from build123d import *

# Parameters (mm, degrees)
SKETCH1_W           = 105
SKETCH1_H           = 4
SKETCH1_W_2         = 2
SKETCH1_H_2         = 9.8
BOSS_EXTRUDE1_DEPTH = 12.5
SKETCH2_W           = 8
SKETCH2_H           = 10
SKETCH2_R           = 1.55
BOSS_EXTRUDE2_DEPTH = 2
SKETCH4_W           = 8
SKETCH4_H           = 10
SKETCH4_R           = 1.55
BOSS_EXTRUDE3_DEPTH = 2
SKETCH5_W           = 101
SKETCH5_H           = 2
CUT_EXTRUDE1_DEPTH  = 1.75
SKETCH6_W           = 101
SKETCH6_H           = 2
CUT_EXTRUDE2_DEPTH  = 1.75


with BuildPart() as part:
    # Sketch1 → Boss-Extrude1 (new body, symmetric)
    with BuildSketch(Plane(origin=(0, 0, 0), x_dir=(0, 0, -1), z_dir=(1, 0, 0))):
        Rectangle(SKETCH1_W, SKETCH1_H)
        Polygon((-52.5, 63.2), (-52.5, 2), (-48.5, 2), (-48.5, 63.2), (-50.5, 63.2), align=None)
        Polygon((48.5, 63.2), (48.5, 2), (52.5, 2), (52.5, 63.2), (50.5, 63.2), align=None)
        with Locations((-49.5, 68.1)):
            Rectangle(SKETCH1_W_2, SKETCH1_H_2)
        with Locations((49.5, 68.1)):
            Rectangle(SKETCH1_W_2, SKETCH1_H_2)
    extrude(amount=BOSS_EXTRUDE1_DEPTH, both=True)

    # Sketch2 → Boss-Extrude2 (add)
    with BuildSketch(Plane.XY.offset(-48.5)):
        with Locations((-16.5, 16)):
            Rectangle(SKETCH2_W, SKETCH2_H)
        with Locations((-16.5, 16)):
            Circle(SKETCH2_R, mode=Mode.SUBTRACT)
        with Locations((-16.5, 44)):
            Rectangle(SKETCH2_W, SKETCH2_H)
        with Locations((-16.5, 44)):
            Circle(SKETCH2_R, mode=Mode.SUBTRACT)
        with Locations((16.5, 16)):
            Rectangle(SKETCH2_W, SKETCH2_H)
        with Locations((16.5, 16)):
            Circle(SKETCH2_R, mode=Mode.SUBTRACT)
        with Locations((16.5, 44)):
            Rectangle(SKETCH2_W, SKETCH2_H)
        with Locations((16.5, 44)):
            Circle(SKETCH2_R, mode=Mode.SUBTRACT)
    extrude(amount=-BOSS_EXTRUDE2_DEPTH)

    # Sketch4 → Boss-Extrude3 (add)
    with BuildSketch(Plane(origin=(0, 0, 48.5), x_dir=(-1, 0, 0), z_dir=(0, 0, -1))):
        with Locations((-16.5, 16)):
            Rectangle(SKETCH4_W, SKETCH4_H)
        with Locations((-16.5, 16)):
            Circle(SKETCH4_R, mode=Mode.SUBTRACT)
        with Locations((-16.5, 44)):
            Rectangle(SKETCH4_W, SKETCH4_H)
        with Locations((-16.5, 44)):
            Circle(SKETCH4_R, mode=Mode.SUBTRACT)
        with Locations((16.5, 16)):
            Rectangle(SKETCH4_W, SKETCH4_H)
        with Locations((16.5, 16)):
            Circle(SKETCH4_R, mode=Mode.SUBTRACT)
        with Locations((16.5, 44)):
            Rectangle(SKETCH4_W, SKETCH4_H)
        with Locations((16.5, 44)):
            Circle(SKETCH4_R, mode=Mode.SUBTRACT)
    extrude(amount=-BOSS_EXTRUDE3_DEPTH)

    # Sketch5 → Cut-Extrude1 (cut)
    with BuildSketch(Plane.ZY.offset(12.5)):
        Polygon((-50.5, 63.2), (-52.5, 63.2), (-52.5, -2), (-50.5, -2), (-50.5, 0), (-50.5, 11), (-50.5, 21), (-50.5, 39), (-50.5, 49), align=None)
        with Locations((0, -1)):
            Rectangle(SKETCH5_W, SKETCH5_H)
        Polygon((50.5, 0), (50.5, -2), (52.5, -2), (52.5, 63.2), (50.5, 63.2), (50.5, 49), (50.5, 39), (50.5, 21), (50.5, 11), align=None)
    extrude(amount=-CUT_EXTRUDE1_DEPTH, mode=Mode.SUBTRACT)

    # Sketch6 → Cut-Extrude2 (cut)
    with BuildSketch(Plane(origin=(12.5, 0, 0), x_dir=(0, 0, -1), z_dir=(1, 0, 0))):
        Polygon((-50.5, 0), (-50.5, 63.2), (-52.5, 63.2), (-52.5, -2), (-50.5, -2), align=None)
        with Locations((0, -1)):
            Rectangle(SKETCH6_W, SKETCH6_H)
        Polygon((50.5, 63.2), (50.5, 0), (50.5, -2), (52.5, -2), (52.5, 63.2), align=None)
    extrude(amount=-CUT_EXTRUDE2_DEPTH, mode=Mode.SUBTRACT)


solid = part.part
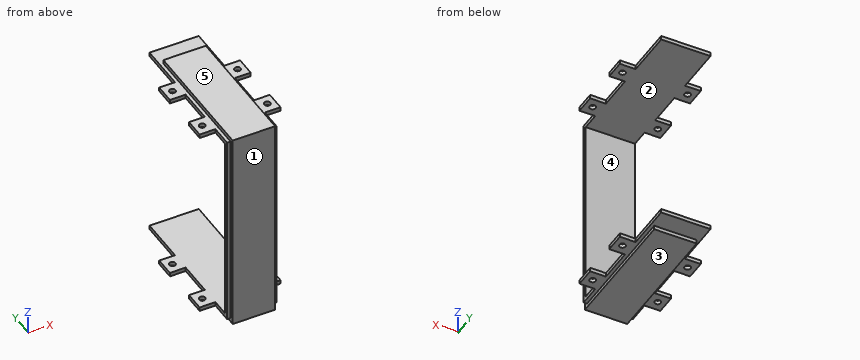
Here's how the part is built. I have some questions about the finished solid (model axes, mm). Face numbers are marked on the shaded views. A direction names the side the tool comes from. Give positions to 0.01 mm unless a question says otherwise; leave off trailing zeros. Loops run counter-clockwise (first coordinate to the right, second up) from the corner with the lowest first, then second, coordinate; pieces in that order, holes last. Notation, with made-up numbers: (43.5, -33.5) -> (84.5, -33.5) arc R17 ccw to (84.5, -0.5) -> close; hole circle Ø10 at (-13, 17.25). An arc over 180 degrees is marked (long way). One line per item, written item: value.
Q1. If I drill on line 1 along Y through (x, z) = (16.5, 49.3); line 2 along Z through (x, y) = (10.5, 28); line 3 along Z through (x, y) = (17, 20), over which ranges is the centre line in solid material (lowest first)?
Answers follow:
line 1: 11 to 14.45, 17.55 to 21, 39 to 42.45, 45.55 to 49
line 2: -52.5 to -48.5, 48.5 to 52.5
line 3: -50.5 to -48.5, 48.5 to 50.5
Q2. Suppose I cut it at C-C on z = 40. Please give me the cut outline in (x, y), then the cut area to 3 significant figures.
Answers follow:
outline: (-12.5, 0) -> (-10.75, 0) -> (-10.75, -2) -> (10.75, -2) -> (10.75, 0) -> (12.5, 0) -> (12.5, 2) -> (-12.5, 2) -> close
area: 93.0 mm^2
Q3. Suppose I cut it at D-D on x = -2. Please give me the cut outline in (y, z).
Answers follow:
outline: (-2, -52.5) -> (63.2, -52.5) -> (63.2, -50.5) -> (73, -50.5) -> (73, -48.5) -> (2, -48.5) -> (2, 48.5) -> (73, 48.5) -> (73, 50.5) -> (63.2, 50.5) -> (63.2, 52.5) -> (-2, 52.5) -> close
Q4. We'd pull the mould along Z, two halves only. Please class the marked faces 1, 2 and 3: pulls with the +Z half, pulls with the -Z half, needs draft (parallel to the pull), parting line crosses it, or undercut.
Answers follow:
face 1: needs draft
face 2: undercut
face 3: pulls with the -Z half
Q5. Suppose I cut it at A-A on x = 16.5. State how many separate pieces and enclosed holes the cut face has, then the cut area to 3 significant figures.
Answers follow:
separate pieces: 8
enclosed holes: 0
area: 55.2 mm^2
Q6. I'm going to push flat-ended pins straight in: pin 1 Ø1 at (y, z) = (58.5, -50) entering from +X; pin 2 Ø1 at (x, z) = (3, -51.5) entering from +Y; pin 3 Ø5 at (x, y) = (-16.5, 44) entering from +Z; pin 4 Ø4 at (x, y) = (16, 30) entering from +Z. Where does each tip first touch, or does it pass through?
Answers follow:
pin 1: x = 12.5
pin 2: y = 63.2
pin 3: z = 50.5
pin 4: through
Q7. On a 3-axis mill with a long thin cutter (end or side, diameter ignored), from which of +Z, -Z, +X, -X, +Y, -Y can I reach the whole of each face in a straight line? I mean the marked faces 4 and 5. Say none if no direction works.
Answers follow:
face 4: +X, -X, +Y
face 5: +Z, +X, -X, +Y, -Y
